from build123d import *

# Parameters (mm, degrees)
F0_W     = 15.7734
F0_H     = 15.7734
F1_DEPTH = 9.6012
F2_R     = 2.4511
F3_DEPTH = 11.43
F4_W     = 13.2842
F4_H     = 13.2842
F4_R     = 3.2258
F5_DEPTH = 7.62
F6_R     = 2.4511
F7_DEPTH = 7.62


# Not quite as in the source:
# - a feature names something its author has since deleted; it is built from what else it names


with BuildPart() as f1:
    # F0 (on Top) → F1 (new body)
    with BuildSketch(Plane.XY):
        Rectangle(F0_W, F0_H)
    extrude(amount=F1_DEPTH)

    # F2 (on face) → F3 (join)
    with BuildSketch(Plane.XY):
        with Locations((-3.94462, 3.9624)):
            Circle(F2_R)
        with Locations((3.9878, 3.9624)):
            Circle(F2_R)
        with Locations((-3.9878, -3.9624)):
            Circle(F2_R)
        with Locations((3.9878, -3.9624)):
            Circle(F2_R)
    extrude(amount=F3_DEPTH)

    # F4 (on face) → F5 (cut)
    with BuildSketch(Plane(origin=(0, 0, 0), x_dir=(1, 0, 0), z_dir=(0, 0, -1))):
        Rectangle(F4_W, F4_H)
        Circle(F4_R, mode=Mode.SUBTRACT)
    extrude(amount=-F5_DEPTH, mode=Mode.SUBTRACT)

    # F6 (on face) → F7 (cut)
    with BuildSketch(Plane(origin=(0, 0, 0), x_dir=(1, 0, 0), z_dir=(0, 0, -1))):
        Circle(F6_R)
    extrude(amount=-F7_DEPTH, mode=Mode.SUBTRACT)


solid = f1.part
Work out the finished part from the listing and answer in its coordinate system (mm). A direction names the side the tool comes from. Round coordinates to 2 decimals unless told otherwise and drop trailing zeros. Loops run counter-clockwise (first coordinate to the right, second up) from the corner with the lowest first, then second, coordinate; pieces in that order, holes last. Notation, with made-up numbers: (33, 82.25) - (90, 82.25) arc R18 cw to (90, 110.25) - close; hole circle Ø4 at (29.5, 3.25). An arc over 180 degrees is marked (long way). One line per item, written item: value.
Q1. Find section A-A on z = 6.25. Give the vertices of the cut face in (x, y), and give its area (3 significant figures).
Check values:
outline: (-7.89, -7.89) - (7.89, -7.89) - (7.89, 7.89) - (-7.89, 7.89) - close; circle Ø6.45 at (0, 0); hole (-6.64, -6.64) - (6.64, -6.64) - (6.64, 6.64) - (-6.64, 6.64) - close; hole circle Ø4.9 at (0, 0)
area: 86.1 mm2
Q2. Find section D-D on x = -3. Give the vertices of the cut face in (y, z), and give its area (3 significant figures).
Check values:
outline: (-7.89, 0) - (-6.64, 0) - (-6.64, 7.62) - (-1.19, 7.62) - (-1.19, 0) - (1.19, 0) - (1.19, 7.62) - (6.64, 7.62) - (6.64, 0) - (7.89, 0) - (7.89, 9.6) - (6.22, 9.6) - (6.22, 11.43) - (1.7, 11.43) - (1.7, 9.6) - (-1.72, 9.6) - (-1.72, 11.43) - (-6.21, 11.43) - (-6.21, 9.6) - (-7.89, 9.6) - close
area: 84.8 mm2
Q3. Straight lines are drawn through the part: probe 1 along Y at (x, z) = (0, 3.5); probe 2 along X at (y, z) = (6.5, 2.5). For each, find the intervals that lie inside material, in ascending order.
Check values:
probe 1: -7.89 to -6.64, -3.23 to -2.45, 2.45 to 3.23, 6.64 to 7.89
probe 2: -7.89 to -6.64, 6.64 to 7.89
Q4. For faces 4 (the flat face through (0, 0, 7.62)), 5 (the cylindrical face through (3.67, -1.53, 10.5)), 6 (the flat face through (-4, -4, 11.43)), determine the directions among +Z, -Z, +X, -X, +Y, -Y from which every point of the face is accessible in a straight line to the end or side of a thin tool.
Check values:
face 4: -Z
face 5: +Z
face 6: +Z, +X, -X, +Y, -Y
Q5. The mould has two halves that part along Y. Classify faces 1 (the cylindrical face through (-1.607, 4.699, 10.503)), 2 (the flat face through (-4, 4, 11.43)), 3 (the flat face through (0, 7.887, 5)): +Y half, -Y half, draft (parallel to the pull), parting line (faces both ways), or undercut.
Check values:
face 1: undercut
face 2: draft
face 3: +Y half
Q6. This flat-tipped pin is pushed along its axis until it touches: pin 1 Ø4.5 at (x, y) = (0, 0) entering from -Z. Where does it stop, or does it pass through?
Check values:
pin 1: z = 7.62
Q7. Find section B-B on x = 0. Give the vertices of the cut face in (y, z), and give its area (3 significant figures).
Check values:
outline: (-7.89, 0) - (-6.64, 0) - (-6.64, 7.62) - (-3.23, 7.62) - (-3.23, 0) - (-2.45, 0) - (-2.45, 7.62) - (2.45, 7.62) - (2.45, 0) - (3.23, 0) - (3.23, 7.62) - (6.64, 7.62) - (6.64, 0) - (7.89, 0) - (7.89, 9.6) - (-7.89, 9.6) - close
area: 62.0 mm2
